```python
from build123d import *

# Parameters (mm, degrees)
SKETCH_1_W                       = 4
SKETCH_1_H                       = 4
EXTRUDE_1_DEPTH                  = 65
FILLET_1_R                       = 1
FILLET_2_R                       = 2
FILLET_3_R                       = 0.5
PATTERN_CIRCULAR_1_COUNT         = 4
FILLET_1_OF_PATTERN_CIRCULAR_1_R = 1
FILLET_2_OF_PATTERN_CIRCULAR_1_R = 2
FILLET_3_OF_PATTERN_CIRCULAR_1_R = 0.5
SKETCH_2_R                       = 3.4
CUT_EXTRUDE_1_DEPTH              = 66
SKETCH_3_R                       = 4.1
CUT_EXTRUDE_2_DEPTH              = 21.7


with BuildPart() as part:
    # 草图1 → 凸台-拉伸1 (new body)
    with BuildSketch(Plane.XY):
        Polygon((5.7, 0), (5.7, 4.427207794), (9.672792206, 8.4), (13.2, 8.4), (13.2, 4.1), (14.1, 4.1), (14.1, 5.1), (15, 5.1), (15, 15), (5.1, 15), (5.1, 14.1), (4.1, 14.1), (4.1, 13.2), (8.4, 13.2), (8.4, 9.672792206), (4.427207794, 5.7), (0, 5.7), (0, 0), align=None)
        with Locations((11.7, 11.7)):
            Rectangle(SKETCH_1_W, SKETCH_1_H, mode=Mode.SUBTRACT)
    extrude_1 = extrude(amount=EXTRUDE_1_DEPTH)

    # 圆角1
    fillet_1_edges = [part.edges().sort_by_distance(p)[0] for p in [
        (13.7, 9.7, 32.5),
        (13.7, 13.7, 32.5),
        (9.7, 13.7, 32.5),
        (9.7, 9.7, 32.5),
    ]]
    fillet(fillet_1_edges, radius=FILLET_1_R)

    # 圆角2
    fillet_2_edges = [part.edges().sort_by_distance(p)[0] for p in [
        (15, 15, 32.5),
    ]]
    fillet(fillet_2_edges, radius=FILLET_2_R)

    # 圆角3
    fillet_3_edges = [part.edges().sort_by_distance(p)[0] for p in [
        (4.427207794, 5.7, 32.5),
        (8.4, 9.672792206, 32.5),
        (8.4, 13.2, 32.5),
        (13.2, 8.4, 32.5),
        (9.672792206, 8.4, 32.5),
        (5.7, 4.427207794, 32.5),
    ]]
    fillet(fillet_3_edges, radius=FILLET_3_R)

    # 阵列(圆周)1: 凸台-拉伸1 ×4 about axis
    pattern_circular_1_axis = Axis((0, 0, 0), (0, 0, 1))
    for i in range(1, PATTERN_CIRCULAR_1_COUNT):
        add(extrude_1.rotate(pattern_circular_1_axis, i * 360 / PATTERN_CIRCULAR_1_COUNT))

    # 圆角1 of 阵列(圆周)1
    fillet_1_of_pattern_circular_1_edges = [part.edges().sort_by_distance(p)[0] for p in [
        (-9.7, 13.7, 32.5),
        (-13.7, 13.7, 32.5),
        (-13.7, 9.7, 32.5),
        (-9.7, 9.7, 32.5),
        (-13.7, -9.7, 32.5),
        (-13.7, -13.7, 32.5),
        (-9.7, -13.7, 32.5),
        (-9.7, -9.7, 32.5),
        (9.7, -13.7, 32.5),
        (13.7, -13.7, 32.5),
        (13.7, -9.7, 32.5),
        (9.7, -9.7, 32.5),
    ]]
    fillet(fillet_1_of_pattern_circular_1_edges, radius=FILLET_1_OF_PATTERN_CIRCULAR_1_R)

    # 圆角2 of 阵列(圆周)1
    fillet_2_of_pattern_circular_1_edges = [part.edges().sort_by_distance(p)[0] for p in [
        (-15, 15, 32.5),
        (-15, -15, 32.5),
        (15, -15, 32.5),
    ]]
    fillet(fillet_2_of_pattern_circular_1_edges, radius=FILLET_2_OF_PATTERN_CIRCULAR_1_R)

    # 圆角3 of 阵列(圆周)1
    fillet_3_of_pattern_circular_1_edges = [part.edges().sort_by_distance(p)[0] for p in [
        (-5.7, 4.427207794, 32.5),
        (-9.672792206, 8.4, 32.5),
        (-13.2, 8.4, 32.5),
        (-8.4, 13.2, 32.5),
        (-8.4, 9.672792206, 32.5),
        (-4.427207794, 5.7, 32.5),
        (-4.427207794, -5.7, 32.5),
        (-8.4, -9.672792206, 32.5),
        (-8.4, -13.2, 32.5),
        (-13.2, -8.4, 32.5),
        (-9.672792206, -8.4, 32.5),
        (-5.7, -4.427207794, 32.5),
        (5.7, -4.427207794, 32.5),
        (9.672792206, -8.4, 32.5),
        (13.2, -8.4, 32.5),
        (8.4, -13.2, 32.5),
        (8.4, -9.672792206, 32.5),
        (4.427207794, -5.7, 32.5),
    ]]
    fillet(fillet_3_of_pattern_circular_1_edges, radius=FILLET_3_OF_PATTERN_CIRCULAR_1_R)

    # 草图2 → 切除-拉伸1 (cut, through all)
    with BuildSketch(Plane.XY.offset(65)):
        Circle(SKETCH_2_R)
    extrude(amount=-CUT_EXTRUDE_1_DEPTH, mode=Mode.SUBTRACT)

    # 草图3 → 切除-拉伸2 (cut, through all)
    with BuildSketch(Plane.ZY.offset(5.7)):
        with Locations((15, 0)):
            Circle(SKETCH_3_R)
    extrude(amount=-CUT_EXTRUDE_2_DEPTH, mode=Mode.SUBTRACT)


solid = part.part
```
Could you check a few things on this model? Use its own coordinates, in mm. A direction names the side the tool comes from. Give positions to 0.01 mm unless a question says otherwise; leave off trailing zeros. Loops run counter-clockwise (first coordinate to the right, second up) from the corner with the lowest first, then second, coordinate; pieces in that order, holes last. Notation, with made-up numbers: (-5.75, 27) - (23.25, 27) arc R21 cw to (23.25, 31) - close; hole circle Ø1 at (78.25, 42.5). An arc over 180 degrees is marked (long way). Answer in a Markdown table with one row per item. Add a question column.
Q1. If we section it at D-D (z = 23): State how many separate pieces and enclosed holes the cut face has, plus the area to 3 significant figures.
Q2. If we section it at C-C (y = 0): List the corners of the cut face in (x, z) for me, plus the area to 3 significant figures.
Q3. We'd pull the mould along X, two halves only. Please class faces 3 (the face through (-15, -9, 32)), 4 (the face through (15, 9, 32)), 5 (the face through (0, 5.7, 32)), 6 (the face through (-9.7, 12, 32)): +X half, -X half, draft (parallel to the pull), parting line (faces both ways), or undercut.
Q4. For pin 1 (4 mm diameter, centred on x = -1, z = 53, fed in from -Y); pin 2 (1 mm diameter, centred on x = 14, z = 45.5, fed in from +Y); pin 3 (0.7 mm diameter, centred on y = -15, z = 22.5, fed in from -X), each with a flat end and sliding along its axis, tell me the tip position at first contact or that it passes through.
Q5. Please list where these lines run through material, in increasing order: L1, parallel to X at y = 12.5, z = 6.5; L2, parallel to X at y = 0, z = 51.5. Write a range as from..to.
Q6. Which directions (+Z, -Z, +X, -X, +Y, -Y) give clear straight access to the entire face, cutting with the end or side of a thin tool? Please do faces 1 (the face through (-13.2, -6, 32)), 2 (the face through (-14.4, 14.43, 32.96)).
Q7. If we section it at A-A (x = 0): List the corners of the cut face in (y, z) for me, plus the area to 3 significant figures.
Q8. If we section it at B-B (x = -12): List the corners of the cut face in (y, z) for me.
The answers:
| question | item | result |
|---|---|---|
| 1 | separate pieces | 1 |
| 1 | enclosed holes | 5 |
| 1 | area | 293 mm^2 |
| 2 | outline | (-5.7, 0) - (-3.4, 0) - (-3.4, 10.9) - (-5.7, 10.9) - close; (-5.7, 19.1) - (-3.4, 19.1) - (-3.4, 65) - (-5.7, 65) - close; (3.4, 0) - (5.7, 0) - (5.7, 10.9) - (3.4, 10.9) - close; (3.4, 19.1) - (5.7, 19.1) - (5.7, 65) - (3.4, 65) - close |
| 2 | area | 261 mm^2 |
| 3 | face 3 | -X half |
| 3 | face 4 | +X half |
| 3 | face 5 | undercut |
| 3 | face 6 | undercut |
| 4 | pin 1 | stops at y = -5.7 |
| 4 | pin 2 | stops at y = 14.94 |
| 4 | pin 3 | stops at x = -14.13 |
| 5 | L1 | x = -15..-13.7, -9.7..-8.4, 8.4..9.7, 13.7..15 |
| 5 | L2 | x = -5.7..-3.4, 3.4..5.7 |
| 6 | face 1 | +Z, -Z |
| 6 | face 2 | +Z, -Z, -X, +Y |
| 7 | outline | (-5.7, 0) - (-3.4, 0) - (-3.4, 12.71) arc R4.1 cw to (-3.4, 17.29) - (-3.4, 65) - (-5.7, 65) - close; (3.4, 0) - (5.7, 0) - (5.7, 65) - (3.4, 65) - (3.4, 17.29) arc R4.1 cw to (3.4, 12.71) - close |
| 7 | area | 295 mm^2 |
| 8 | outline | (-15, 0) - (-13.7, 0) - (-13.7, 65) - (-15, 65) - close; (-9.7, 0) - (-8.4, 0) - (-8.4, 65) - (-9.7, 65) - close; (8.4, 0) - (9.7, 0) - (9.7, 65) - (8.4, 65) - close; (13.7, 0) - (15, 0) - (15, 65) - (13.7, 65) - close |
